Read the model definition and answer for the solid it produces. Units are mm, in the model's axes. A direction names the side the tool comes from. Give positions to 0.01 mm unless a question says otherwise; leave off trailing zeros. Write each loop counter-clockwise with the first axis right and the second up, starting at its lowest first coordinate (ties: lowest second). Pieces come first, ordered by that corner, then holes. Notation, with made-up numbers: M 52,61.5 L 66,61.5 A26 ccw 66,79.5 Z; hole C 81,15 d9. An arc over 180 degrees is marked long. Use a Markdown table: item, result. Add a question column.
Item 1: Consider probe 1 along Y at (x, z) = (0, -3.05); probe 2 along X at (y, z) = (0, 10.5); probe 3 along X at (y, z) = (-0.5, 8.5). Determine where each line is inside the solid, lowest interval first. Write a range as [from, to].
Item 2: A cutting plane is placed at A-A on z = -4. Determine the outline of the cut face in (x, y), then the cut area to 3 significant figures.
Item 3: For faces 4 (the flat face through (12.37, -7.44, -2.96)), 5 (the cylindrical face through (-0.585, -2.636, -3.788)), determine the directions among +Z, -Z, +X, -X, +Y, -Y from which every point of the face is accessible in a straight line to the end or side of a thin tool.
Item 4: Given P1, Ø1.8, axis at x = -1, y = 0.5, coming from the +Z side; P2, Ø5, axis at x = 9, y = 8.5, coming from the +Z side; P3, Ø2, axis at x = 14, z = -5, coming from the -Y side, each flat-ended and moving along its own axis, determine where each tip first touches the part or whether it passes through.
Item 5: The mould has two halves that part along X. Classify faces 1 (the flat face through (0.255, 10.264, 5.2)), 2 (the cylindrical face through (-3, 0, 6)), 3 (the cylindrical face through (0.059, -24.867, -2.848)): pulls with the +X half, pulls with the -X half, needs draft (parallel to the pull), parting line crosses it, or undercut.
from build123d import *

# Parameters (mm, degrees)
F4_R          = 5
F9_DEPTH      = 10
F10_T1_DEPTH  = 23.3205080757
F10_T3_DEPTH  = 36.1435935394
F10_T5_DEPTH  = 36.1435935394
F10_T7_DEPTH  = 36.1435935394
F10_T12_DEPTH = 4
F10_T18_DEPTH = 4
F10_T24_DEPTH = 4
F6_R          = 2.7
F11_DEPTH     = 8
F8_R          = 3
F12_DEPTH     = 25
F13_R         = 2.5


# Not quite as in the source:
# - a fillet or chamfer that OpenCascade refuses, or shapes differently, is made with other operations: its cross-section is extruded or revolved along the edge and cut away or added


with BuildPart() as f3:
    # F0 (on Top) → F3 section 0
    with BuildSketch(Plane.XY, mode=Mode.PRIVATE) as f3_s0:
        Polygon((25, 14.4337567297), (-25, 14.4337567297), (0, -28.8675134595), align=None)
    loft([f3_s0.sketch, Vertex(0, 0, 18)])

    # F4
    f4_edges = [f3.edges().sort_by_distance(p)[0] for p in [
        (12.5, 7.216878, 9),
        (0, -14.433757, 9),
        (-12.5, 7.216878, 9),
    ]]
    fillet(f4_edges, radius=F4_R)

    # F0 (on Top) → F9 (join)
    with BuildSketch(Plane.XY):
        Polygon((25, 14.4337567297), (-25, 14.4337567297), (0, -28.8675134595), align=None)
    extrude(amount=-F9_DEPTH)

    # F10: fillet of radius 4 on 6 edges, made by hand

    # F10_s2 → F10_t1 (cut)
    with BuildSketch(Plane.XY.offset(-6)):
        with BuildLine():
            ThreePointArc((21.5358983849, 8.4337567297), (21.5358983849, 12.4337567297), (18.0717967697, 14.4337567297))
            Line((18.0717967697, 14.4337567297), (25, 14.4337567297))
            Line((25, 14.4337567297), (21.5358983849, 8.4337567297))
        make_face()
        with BuildLine():
            ThreePointArc((-21.5358983849, 8.4337567297), (-21.5358983849, 12.4337567297), (-18.0717967697, 14.4337567297))
            Line((-18.0717967697, 14.4337567297), (-25, 14.4337567297))
            Line((-25, 14.4337567297), (-21.5358983849, 8.4337567297))
        make_face()
        with BuildLine():
            ThreePointArc((3.4641016151, -22.8675134595), (0, -24.8675134595), (-3.4641016151, -22.8675134595))
            Line((-3.4641016151, -22.8675134595), (0, -28.8675134595))
            Line((0, -28.8675134595), (3.4641016151, -22.8675134595))
        make_face()
    extrude(amount=F10_T1_DEPTH, mode=Mode.SUBTRACT)

    # F10_s4 → F10_t3 (cut)
    with BuildSketch(Plane.YZ.offset(-18.0717967697)):
        with BuildLine():
            ThreePointArc((14.4337567297, -6), (13.2621838545, -8.8284271247), (10.4337567297, -10))
            Line((10.4337567297, -10), (14.4337567297, -10))
            Line((14.4337567297, -10), (14.4337567297, -6))
        make_face()
    extrude(amount=F10_T3_DEPTH, mode=Mode.SUBTRACT)

    # F10_s6 → F10_t5 (cut)
    with BuildSketch(Plane(origin=(-9.0358983849, 15.6506350946, 0), x_dir=(0, 0, 1), z_dir=(0.5, -0.8660254038, 0))):
        with BuildLine():
            ThreePointArc((-6, 14.4337567297), (-8.8284271247, 13.2621838545), (-10, 10.4337567297))
            Line((-10, 10.4337567297), (-10, 14.4337567297))
            Line((-10, 14.4337567297), (-6, 14.4337567297))
        make_face()
    extrude(amount=F10_T5_DEPTH, mode=Mode.SUBTRACT)

    # F10_s8 → F10_t7 (cut)
    with BuildSketch(Plane(origin=(-9.0358983849, -15.6506350946, 0), x_dir=(0, 0, 1), z_dir=(0.5, 0.8660254038, 0))):
        with BuildLine():
            ThreePointArc((-6, 14.4337567297), (-8.8284271247, 13.2621838545), (-10, 10.4337567297))
            Line((-10, 10.4337567297), (-10, 14.4337567297))
            Line((-10, 14.4337567297), (-6, 14.4337567297))
        make_face()
    extrude(amount=F10_T7_DEPTH, mode=Mode.SUBTRACT)


with BuildPart() as f10_tool10:
    # F10_s11 → F10_t12 (new body)
    with BuildSketch(Plane.XY.offset(-6)):
        Polygon((18.0717967697, 10.4337567297), (21.5358983849, 8.4337567297), (25, 14.4337567297), (18.0717967697, 14.4337567297), align=None)
    extrude(amount=-F10_T12_DEPTH)

    # F10_s13 → F10_t14 (revolve, cut)
    with BuildSketch(Plane(origin=(18.0717967697, 10.4337567297, -6), x_dir=(-0.8660254038, -0.5, 0), z_dir=(0.5, -0.8660254038, 0))):
        with BuildLine():
            ThreePointArc((0, -4), (4, 0), (0, 4))
            Line((0, 4), (0, -4))
        make_face()
    revolve(axis=Axis((18.0717967697, 10.4337567297, -6), (0, 0, -1)), mode=Mode.SUBTRACT)


with BuildPart() as f3_1:
    add(f3.part)

    # F10_t9: cut F10_tool10
    add(f10_tool10.part, mode=Mode.SUBTRACT)


with BuildPart() as f10_tool16:
    # F10_s17 → F10_t18 (new body)
    with BuildSketch(Plane.XY.offset(-6)):
        Polygon((-18.0717967697, 10.4337567297), (-21.5358983849, 8.4337567297), (-25, 14.4337567297), (-18.0717967697, 14.4337567297), align=None)
    extrude(amount=-F10_T18_DEPTH)

    # F10_s19 → F10_t20 (revolve, cut)
    with BuildSketch(Plane(origin=(-18.0717967697, 10.4337567297, -6), x_dir=(0.8660254038, -0.5, 0), z_dir=(0.5, 0.8660254038, 0))):
        with BuildLine():
            ThreePointArc((0, -4), (4, 0), (0, 4))
            Line((0, 4), (0, -4))
        make_face()
    revolve(axis=Axis((-18.0717967697, 10.4337567297, -6), (0, 0, -1)), mode=Mode.SUBTRACT)


with BuildPart() as f3_2:
    add(f3_1.part)

    # F10_t15: cut F10_tool16
    add(f10_tool16.part, mode=Mode.SUBTRACT)


with BuildPart() as f10_tool22:
    # F10_s23 → F10_t24 (new body)
    with BuildSketch(Plane.XY.offset(-6)):
        Polygon((0, -20.8675134595), (3.4641016151, -22.8675134595), (0, -28.8675134595), (-3.4641016151, -22.8675134595), align=None)
    extrude(amount=-F10_T24_DEPTH)

    # F10_s25 → F10_t26 (revolve, cut)
    with BuildSketch(Plane(origin=(0, -20.8675134595, -6), x_dir=(0, 1, 0), z_dir=(-1, 0, 0))):
        with BuildLine():
            ThreePointArc((0, -4), (4, 0), (0, 4))
            Line((0, 4), (0, -4))
        make_face()
    revolve(axis=Axis((0, -20.8675134595, -6), (0, 0, -1)), mode=Mode.SUBTRACT)


with BuildPart() as f3_3:
    add(f3_2.part)

    # F10_t21: cut F10_tool22
    add(f10_tool22.part, mode=Mode.SUBTRACT)

    # F6 (on offset) → F11 (cut)
    with BuildSketch(Plane.XY.offset(-9)):
        Circle(F6_R)
    extrude(amount=F11_DEPTH, mode=Mode.SUBTRACT)

    # F8 (on offset) → F12 (cut)
    with BuildSketch(Plane.XY.offset(-1)):
        Circle(F8_R)
    extrude(amount=F12_DEPTH, mode=Mode.SUBTRACT)

    # F13
    f13_edges = [f3_3.edges().sort_by_distance(p)[0] for p in [
        (-2.7, 0, -9),
    ]]
    fillet(f13_edges, radius=F13_R)


solid = f3_3.part
Filled in:
| question | item | result |
|---|---|---|
| 1 | probe 1 | [-24.87, -2.7], [2.7, 14.43] |
| 1 | probe 2 | [-6.94, -3], [3, 6.94] |
| 1 | probe 3 | [-8.51, -2.96], [2.96, 8.51] |
| 2 | outline | M -21.54,8.43 L -3.46,-22.87 A4 ccw 3.46,-22.87 L 21.54,8.43 A4 ccw 18.07,14.43 L -18.07,14.43 A4 ccw Z; hole C 0,0 d5.4 |
| 2 | area | 1,030 mm² |
| 3 | face 4 | +Z, -Z, +X, -Y |
| 3 | face 5 | +Z |
| 4 | P1 | z = -8.22 |
| 4 | P2 | z = 9.43 |
| 4 | P3 | y = -6.35 |
| 5 | face 1 | needs draft |
| 5 | face 2 | undercut |
| 5 | face 3 | parting line crosses it |
